The model under review builds one solid part; all positions refer to its coordinate system, in mm. Face numbers are marked on the shaded views. A direction names the side the tool comes from. Round coordinates to 2 decimals unless told otherwise and drop trailing zeros. Loops run counter-clockwise (first coordinate to the right, second up) from the corner with the lowest first, then second, coordinate; pieces in that order, holes last. Notation, with made-up numbers: M 5.5,-8 L 9.5,-8 A18 cw 9.5,27 Z; hole C 40,-14.75 d9. An arc over 180 degrees is marked long. Use a Markdown table: item, result. Add a question column.
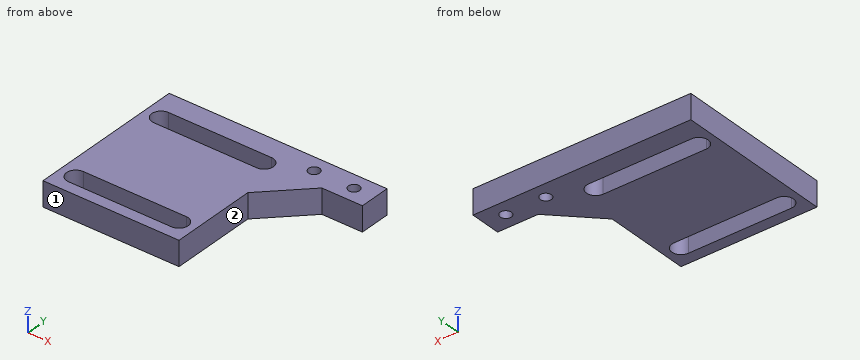
```python
from build123d import *

# Parameters (mm, degrees)
SKETCH7_R           = 1.35
BOSS_EXTRUDE4_DEPTH = 6
CHAMFER1_SIZE       = 10


with BuildPart() as part:
    # Sketch7 → Boss-Extrude4 (new body)
    with BuildSketch(Plane.XY):
        Polygon((-52.845, 0), (0, 0), (0, -7.5), (-19.845, -7.5), (-19.845, -38.5), (-52.845, -38.5), align=None)
        with Locations((-14.69, -3.75)):
            Circle(SKETCH7_R, mode=Mode.SUBTRACT)
        with Locations((-5, -3.75)):
            Circle(SKETCH7_R, mode=Mode.SUBTRACT)
        with BuildLine():
            Line((-48.845, -5.25), (-23.845, -5.25))
            ThreePointArc((-23.845, -5.25), (-21.595, -7.5), (-23.845, -9.75))
            Line((-23.845, -9.75), (-48.845, -9.75))
            ThreePointArc((-48.845, -9.75), (-51.095, -7.5), (-48.845, -5.25))
        make_face(mode=Mode.SUBTRACT)
        with BuildLine():
            Line((-48.845, -31.25), (-23.845, -31.25))
            ThreePointArc((-23.845, -31.25), (-21.595, -33.5), (-23.845, -35.75))
            Line((-23.845, -35.75), (-48.845, -35.75))
            ThreePointArc((-48.845, -35.75), (-51.095, -33.5), (-48.845, -31.25))
        make_face(mode=Mode.SUBTRACT)
    extrude(amount=BOSS_EXTRUDE4_DEPTH)

    # Chamfer1
    chamfer1_edges = [part.edges().sort_by_distance(p)[0] for p in [
        (-19.845, -7.5, 3),
    ]]
    chamfer(chamfer1_edges, length=CHAMFER1_SIZE)


solid = part.part
```
(1) Consider section B-B, the plane x = -5. Give the boundary of the cut face in (y, z).
(2) Insertion check: pin 1 Ø6 at (x, y) = (-18, -11.5) entering from -Z; pin 2 Ø2 at (y, z) = (-33, 2.5) entering from +X (3 decimals). Each pin has a flat end and moves straight along its axis. Give the tip position at first contact, or say it passes through.
(3) For the marked faces 1 and 2, list the 3-axis set-ups (+Z, -Z, +X, -X, +Y, -Y) from which the entire face can be reached by the end or side of a thin tool; tool diameter is ignored.
(4) To check wall thickness, follow probe 1 along Y at (x, z) = (-40, 4.9); probe 2 along Y at (x, z) = (-50, 5.5); probe 3 along X at (y, z) = (-31, 5.6) (3 decimals). State the ranges of each line that lie inside material, in increasing order.
(5) Consider section A-A, the plane y = -3.75. Give the boundary of the cut face in (x, z) (3 decimals).
(6) Consider section C-C, the plane z = 3.85. Give the boundary of the cut face in (x, y) (3 decimals).
(7) Consider section D-D, the plane x = -41. Give the boundary of the cut face in (y, z), then the cut area to 3 significant figures.
Found:
| question | item | result |
|---|---|---|
| 1 | outline | M -7.5,0 L -5.1,0 L -5.1,6 L -7.5,6 Z; M -2.4,0 L 0,0 L 0,6 L -2.4,6 Z |
| 2 | pin 1 | stops at z = 0 |
| 2 | pin 2 | stops at x = -19.845 |
| 3 | face 1 | +Z, -Z, +X, -X, -Y |
| 3 | face 2 | +Z, -Z, +X, -Y |
| 4 | probe 1 | y = -38.5 to -35.75, -31.25 to -9.75, -5.25 to 0 |
| 4 | probe 2 | y = -38.5 to -35.43, -31.57 to -9.43, -5.57 to 0 |
| 4 | probe 3 | x = -52.845 to -19.845 |
| 5 | outline | M -52.845,0 L -16.04,0 L -16.04,6 L -52.845,6 Z; M -13.34,0 L -6.35,0 L -6.35,6 L -13.34,6 Z; M -3.65,0 L 0,0 L 0,6 L -3.65,6 Z |
| 6 | outline | M -52.845,-38.5 L -19.845,-38.5 L -19.845,-17.5 L -9.845,-7.5 L 0,-7.5 L 0,0 L -52.845,0 Z; hole M -48.845,-35.75 L -23.845,-35.75 A2.25 ccw -23.845,-31.25 L -48.845,-31.25 A2.25 ccw Z; hole M -48.845,-9.75 L -23.845,-9.75 A2.25 ccw -23.845,-5.25 L -48.845,-5.25 A2.25 ccw Z; hole C -14.69,-3.75 d2.7; hole C -5,-3.75 d2.7 |
| 7 | outline | M -38.5,0 L -35.75,0 L -35.75,6 L -38.5,6 Z; M -31.25,0 L -9.75,0 L -9.75,6 L -31.25,6 Z; M -5.25,0 L 0,0 L 0,6 L -5.25,6 Z |
| 7 | area | 177 mm^2 |
